The model under review builds one solid part; all positions refer to its coordinate system, in mm. Face numbers are marked on the shaded views. A direction names the side the tool comes from. Round coordinates to 2 decimals unless told otherwise and drop trailing zeros. Write each loop counter-clockwise with the first axis right and the second up, starting at its lowest first coordinate (ties: lowest second). Pieces come first, ordered by that corner, then holes.
Item 1: Add section C-C (y = 30.5). Give the boundary of the cut face in (x, z), plus the area to 3 significant figures.
Item 2: Add section B-B (z = -13.5). Give the boundary of the cut face in (x, y), plus the area to 3 significant figures.
Item 3: Add section D-D (x = 35). Give the boundary of the cut face in (y, z).
Item 4: Clearance check with flat-ended pins moving along their axes: pin 1 Ø12 at (x, y) = (35, 61.5) entering from +Z; pin 2 Ø1.5 at (y, z) = (10.5, -10) entering from +X; pin 3 Ø1 at (x, y) = (35, 8) entering from -Z. State where each tip first meets the part, or that it passes through.
Item 5: Machinability: for the marked faces 4, 5, 6 and 7, which of the approach directions +Z, -Z, +X, -X, +Y, -Y give a long, thin tool a straight path to every point of the face, cutting with its end or side? Answer none if there is none.
Item 6: To check wall thickness, follow L1, parallel to X at y = 67.25, z = -22.5; L2, parallel to Z at x = 22, y = 42; L3, parallel to X at y = 42.5, z = -22. State the ranges of each line that lie inside material, in increasing order.
Item 7: Add section A-A (x = 26). Give the boundary of the cut face in (y, z).
Item 8: Draft analysis for pull direction X (two halves, no side actions). For the marked faces 1, 2 and 3, state which applies: +X half, -X half, draft (parallel to the pull), parting line (faces both ways), or undercut.
Autodesk Inventor part; units mm, degrees
ref_plane "YZ Plane" through (0, 0, 0) normal (1, 0, 0) x (0, 1, 0)
ref_plane "XZ Plane" through (0, 0, 0) normal (0, 1, 0) x (-1, 0, 0)
ref_plane "XY Plane" through (0, 0, 0) normal (0, 0, 1) x (1, 0, 0)
sketch "Sketch1" plane through (0, 0, 0) normal (0, 1, 0) x (-1, 0, 0)
  line L0 (0, 0) -> (0, -45)
  line L1 (0, -45) -> (-45, -45)
  line L2 (-45, -45) -> (-45, 0)
  line L3 (-45, 0) -> (0, 0)
  dimension "d0" = 45
  dimension "d1" = 45
  dimension "d2" = 45
extrude "Extrusion1" add sketch "Sketch1" along normal blind 6
sketch "Sketch2" plane through (0, 6, 0) normal (0, 1, 0) x (1, 0, 0)
  line L0 (0, 0) -> (0, 22.5)
  line L1 (0, 45) -> (0, 0)
  line L2 (0, 22.5) -> (22.5, 22.5)
  circle A0 centre (22.5, 22.5) radius 22.5
  dimension "d5" = 22.5
  dimension "d6" = 22.5
  dimension "d7" = 45
extrude "Extrusion2" add sketch "Sketch2" along normal blind 63.5
sketch "Sketch3" plane through (0, 0, 0) normal (0, -1, 0) x (1, 0, 0)
  line L0 (0, -45) -> (0, 0)
  line L1 (0, 0) -> (0, -22.5)
  circle A0 centre (22.5, -22.5) radius 18.25
  dimension "d12" = 36.5
extrude "Extrusion3" cut sketch "Sketch3" against normal blind 65
sketch "Sketch4" plane through (22.5, 69.5, -22.5) normal (0, 1, 0) x (1, 0, 0)
  circle A0 centre (0, 0) radius 6.75
  point P0 (-22.5, -22.5)
  dimension "d15" = 13.5
extrude "Extrusion4" cut sketch "Sketch4" against normal blind 4.5
sketch "Sketch5" plane through (0, 0, 0) normal (0, -1, 0) x (1, 0, 0)
  line L0 (0, -45) -> (0, 0)
  line L1 (0, 0) -> (22.5, 0)
  line L2 (0, 0) -> (45, 0)
sketch "Sketch6" plane through (22.5, 65, -22.5) normal (0, -1, 0) x (1, 0, 0)
  point P0 (-22.5, 22.5)
properties part number "MotorSupport"
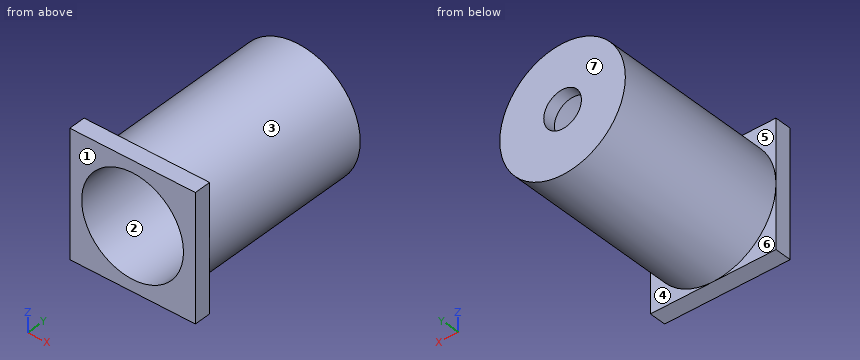
Numbers:
1. outline: circle Ø45 at (22.5, -22.5); hole circle Ø36.5 at (22.5, -22.5)
1. area: 544 mm2
2. outline: (0, 0) - (6.62, 0) - (6.62, 65) - (38.38, 65) - (38.38, 0) - (45, 0) - (45, 6) - (43.12, 6) - (43.12, 69.5) - (1.88, 69.5) - (1.88, 6) - (0, 6) - close
2. area: 825 mm2
3. outline: (0, -45) - (6, -45) - (6, -41.21) - (69.5, -41.21) - (69.5, -3.79) - (6, -3.79) - (6, 0) - (0, 0) - (0, -9.2) - (65, -9.2) - (65, -35.8) - (0, -35.8) - close
4. pin 1: stops at z = -0.96
4. pin 2: stops at x = 41.69
4. pin 3: stops at z = -41.53
5. face 4: -Z, +X, +Y
5. face 5: +Z, -X, +Y
5. face 6: -Z, -X, +Y
5. face 7: +Z, -Z, +X, -X, +Y
6. L1: x = 0 to 15.75, 29.25 to 45
6. L2: z = -44.99 to -40.74, -4.26 to -0.01
6. L3: x = 0.01 to 4.26, 40.74 to 44.99
7. outline: (0, -45) - (6, -45) - (6, -44.73) - (69.5, -44.73) - (69.5, -28.27) - (65, -28.27) - (65, -40.41) - (0, -40.41) - close; (0, -4.59) - (65, -4.59) - (65, -16.73) - (69.5, -16.73) - (69.5, -0.27) - (6, -0.27) - (6, 0) - (0, 0) - close
8. face 1: draft
8. face 2: undercut
8. face 3: parting line
